Geometry: final body of the model. Coordinates: model frame, mm. Give positions to 0.01 mm unless a question says otherwise; leave off trailing zeros. Order: outer loops, then holes, each group sorted by start corner. A loop starts at its lowest first (then second) coordinate and runs counter-clockwise, first axis right, second up. Notation, with made-up numbers: (-11.5, 36) -> (38.5, 36) arc R16 ccw to (38.5, 40) -> close; hole circle Ø7 at (82.5, -4). An arc over 180 degrees is marked (long way). One line per question, with ' | ' between items.
from build123d import *

# Parameters (mm, degrees)
SKETCH1_R           = 51.5
SKETCH1_R_2         = 33
BOSS_EXTRUDE1_DEPTH = 59.5
SKETCH2_W           = 5.951131742
SKETCH2_H           = 4.923958597
BOSS_EXTRUDE2_DEPTH = 50
CIRPATTERN1_COUNT   = 30


with BuildPart() as part:
    # Sketch1 → Boss-Extrude1 (new, symmetric)
    with BuildSketch(Plane.XY):
        Circle(SKETCH1_R)
        Circle(SKETCH1_R_2, mode=Mode.SUBTRACT)
    extrude(amount=BOSS_EXTRUDE1_DEPTH, both=True)

    # Sketch2 → Boss-Extrude2 (add, symmetric)
    with BuildSketch(Plane.XY):
        with Locations((0, -35.327554111)):
            Rectangle(SKETCH2_W, SKETCH2_H)
    boss_extrude2 = extrude(amount=BOSS_EXTRUDE2_DEPTH, both=True)

    # CirPattern1: Boss-Extrude2 ×30 about axis
    cirpattern1_axis = Axis((0, 0, 0), (0, 0, 1))
    for i in range(1, CIRPATTERN1_COUNT):
        add(boss_extrude2.rotate(cirpattern1_axis, i * 360 / CIRPATTERN1_COUNT))


solid = part.part
1) Pull-direction query (X, two-part tool) for faces 1 (the flat face through (-31.27, -10.12, 0.7)), 2 (the flat face through (13.406, 30.007, 0.7)), 3 (the flat face through (-1, -34, 59.5)); classes: +X half, -X half, draft (parallel to the pull), parting line (faces both ways), or undercut.
Check result:
face 1: undercut | face 2: undercut | face 3: draft
2) Section B-B on y = -17. Return loops of the section in (x, z).
Check result:
outline: (-48.61, -59.5) -> (-28.28, -59.5) -> (-28.28, -50) -> (-28.13, -50) -> (-28.13, 50) -> (-28.28, 50) -> (-28.28, 59.5) -> (-48.61, 59.5) -> close; (28.13, -50) -> (28.28, -50) -> (28.28, -59.5) -> (48.61, -59.5) -> (48.61, 59.5) -> (28.28, 59.5) -> (28.28, 50) -> (28.13, 50) -> close
3) Material intervals for probe 1 along Y at (x, z) = (0, -4); probe 2 along X at (y, z) = (2, 47); probe 3 along Y at (x, z) = (-3.5, -12), sorted ascending. Write a range as from..to.
Check result:
probe 1: y = -51.5..-32.87, 32.87..51.5 | probe 2: x = -51.46..-32.84, 32.84..51.46 | probe 3: y = -51.38..-32.81, 32.81..51.38
4) Section A-A on x = 0. Return loops of the section in (y, z), plus the area to 3 significant figures.
Check result:
outline: (-51.5, -59.5) -> (-33, -59.5) -> (-33, -50) -> (-32.87, -50) -> (-32.87, 50) -> (-33, 50) -> (-33, 59.5) -> (-51.5, 59.5) -> close; (32.87, -50) -> (33, -50) -> (33, -59.5) -> (51.5, -59.5) -> (51.5, 59.5) -> (33, 59.5) -> (33, 50) -> (32.87, 50) -> close | area: 4,430 mm^2
5) Contact query for flat-ended pins moving along their axis: pin 1 Ø6 at (x, z) = (41, -20.5) entering from -Y; pin 2 Ø1 at (y, z) = (19.5, 39) entering from +X; pin 3 Ø5 at (x, z) = (1, 16.5) entering from -Y. Output: stop coordinate, or through.
Check result:
pin 1: stops at y = -34.76 | pin 2: stops at x = 47.87 | pin 3: stops at y = -51.5
